from build123d import *

# Parameters (mm, degrees)
SKETCH1_W           = 18
SKETCH1_H           = 6
SKETCH1_R           = 1.5
BOSS_EXTRUDE1_DEPTH = 3
SKETCH2_W           = 5
SKETCH2_H           = 1.5
CUT_EXTRUDE1_DEPTH  = 12.22497216


with BuildPart() as part:
    # Sketch1 → Boss-Extrude1 (new body)
    with BuildSketch(Plane(origin=(0, 0, 0), x_dir=(1, 0, 0), z_dir=(0, 1, 0))):
        Rectangle(SKETCH1_W, SKETCH1_H)
        with Locations(Location((-6.5, 0, 0), (0, 0, 270))):
            Circle(SKETCH1_R, mode=Mode.SUBTRACT)
        with Locations(Location((6.5, 0, 0), (0, 0, 270))):
            Circle(SKETCH1_R, mode=Mode.SUBTRACT)
    extrude(amount=BOSS_EXTRUDE1_DEPTH)

    # Sketch2 → Cut-Extrude1 (cut, through all)
    with BuildSketch(Plane.XY.offset(3)):
        with Locations((0, 0.75)):
            Rectangle(SKETCH2_W, SKETCH2_H)
    extrude(amount=-CUT_EXTRUDE1_DEPTH, mode=Mode.SUBTRACT)


solid = part.part
Geometry check sheet. Reference: the model listing, model coordinates, mm. A direction names the side the tool comes from. Give positions to 0.01 mm unless a question says otherwise; leave off trailing zeros. Loops run counter-clockwise (first coordinate to the right, second up) from the corner with the lowest first, then second, coordinate; pieces in that order, holes last. Notation, with made-up numbers: M 41,-6.5 L 66,-6.5 A19 ccw 66,19.5 Z; hole C -22.5,78.5 d11. An arc over 180 degrees is marked long. Answer as a JSON object with one key per item and string values. Group by question number.
Item 1: Sectioned sample at D-D on y = 2.5. Record the boundary of the cut face in (x, z).
Item 2: Mould release check, pull along Z, two halves, no side actions. Record for faces 3 (the flat face through (0, 3, 0)), 4 (the cylindrical face through (-8, 1, 0)), 5 (the flat face through (0, 2, -3)): pulls with the +Z half, pulls with the -Z half, needs draft (parallel to the pull), parting line crosses it, or undercut.
Item 3: Material ranges on L1, parallel to X at y = 1.1, z = 0; L2, parallel to X at y = 1.2, z = -2.5; L3, parallel to X at y = 2.3, z = 0, recorded low to high.
Item 4: Sectioned sample at A-A on x = 6.5. Record the boundary of the cut face in (y, z), plus the area to 3 significant figures.
Item 5: Sectioned sample at B-B on z = 0. Record the boundary of the cut face in (x, y).
Item 6: Access from +Z, -Z, +X, -X, +Y, -Y to the whole of each face (thin tool, end or side, straight path). Record for faces 1 (the flat face through (-2.5, 1, 0)), 2 (the cylindrical face through (5, 1, 0)).
Item 7: Gauge pin test, flat end, axial feed: pin 1 (1.5 mm diameter, centred on x = -0.5, z = -0.5, fed in from -Y). Record the tip position at first contact, or that the pin passes through.
Item 8: Sectioned sample at C-C on y = 0.7. Record the boundary of the cut face in (x, z), plus the area to 3 significant figures.
Findings below:
{
 "1": {"outline": "M -9,-3 L 9,-3 L 9,3 L -9,3 Z; hole C -6.5,0 d3; hole C 6.5,0 d3"},
 "2": {"face 3": "needs draft", "face 4": "undercut", "face 5": "pulls with the -Z half"},
 "3": {"L1": "-9 to -8, -5 to -2.5, 2.5 to 5, 8 to 9", "L2": "-9 to -2.5, 2.5 to 9", "L3": "-9 to -8, -5 to 5, 8 to 9"},
 "4": {"outline": "M 0,-3 L 3,-3 L 3,-1.5 L 0,-1.5 Z; M 0,1.5 L 3,1.5 L 3,3 L 0,3 Z", "area": "9.00 mm2"},
 "5": {"outline": "M -9,0 L -8,0 L -8,3 L -9,3 Z; M -5,0 L -2.5,0 L -2.5,1.5 L 2.5,1.5 L 2.5,0 L 5,0 L 5,3 L -5,3 Z; M 8,0 L 9,0 L 9,3 L 8,3 Z"},
 "6": {"face 1": "+Z, -Z, -Y", "face 2": "+Y, -Y"},
 "7": {"pin 1": "y = 1.5"},
 "8": {"outline": "M -9,-3 L -2.5,-3 L -2.5,3 L -9,3 Z; M 2.5,-3 L 9,-3 L 9,3 L 2.5,3 Z; hole C -6.5,0 d3; hole C 6.5,0 d3", "area": "63.9 mm2"}
}
